Study the drawing (mm; zero at the part's minimum x, y, z) and answer. A direction names the side the tool comes from. Coordinates: 2 decimals unless noted, no trailing zeros. Write each loop counter-clockwise with the first axis right and the second up, starting at its lowest first coordinate (ties: lowest second). Pieces come first, ordered by that corner, then holes. Notation, with made-up numbers: (-14, 35.25) -> (6, 35.25) arc R21 cw to (6, 66.25) -> close; hole circle Ø2 at (37, 63.5). An arc over 180 degrees is marked (long way). Answer in a Markdown table with one row per item. Add a question column.
Item 1: Section B-B on z = 127 is taken. Write down the section's boundary in (x, y).
Item 2: Straight lines are drawn through the part: line 1 (Z direction, x = 6.5, y = 74); line 2 (Y direction, x = 48.5, z = 130). For each, find the intervals that lie inside material, in ascending order. Write a range as from..to.
Item 3: Section A-A on y = 45.5 is taken. Write down the section's boundary in (x, z), then the cut area to 3 significant figures.
Item 4: Which of the six approach directions +Z, -Z, +X, -X, +Y, -Y give full straight-line access (tool end or side, diameter ignored) to the marked faces 1, 2 and 3?
Item 5: Given pin 1 Ø6 at (y, z) = (39.5, 76) entering from -X; pin 2 Ø8 at (x, z) = (52, 139) entering from +Y, each flat-ended and moving along its own axis, determine where each tip first touches the part or whether it passes through.
Item 6: Section D-D on y = 57.5 is taken. Write down the section's boundary in (x, z), then the cut area to 3 significant figures.
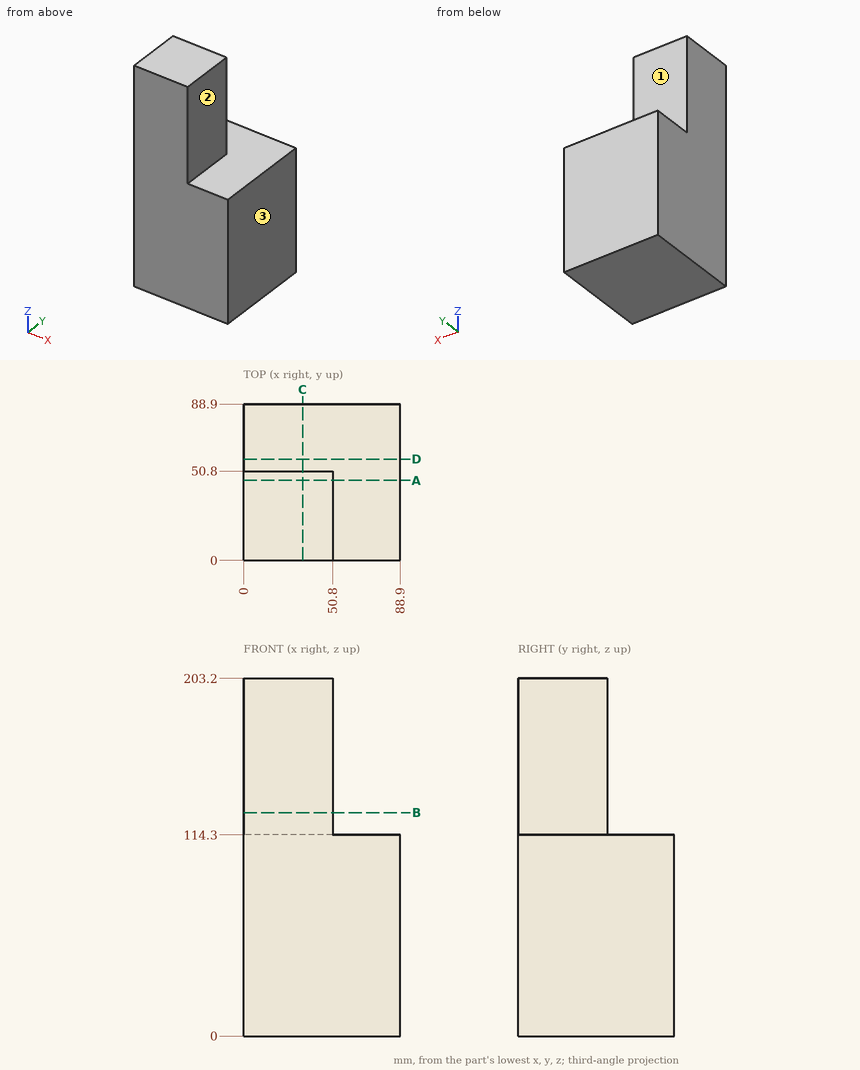
Results below:
| question | item | result |
|---|---|---|
| 1 | outline | (0, 0) -> (50.8, 0) -> (50.8, 50.8) -> (0, 50.8) -> close |
| 2 | line 1 | z = 0..114.3 |
| 2 | line 2 | y = 0..50.8 |
| 3 | outline | (0, 0) -> (88.9, 0) -> (88.9, 114.3) -> (50.8, 114.3) -> (50.8, 203.2) -> (0, 203.2) -> close |
| 3 | area | 14,700 mm2 |
| 4 | face 1 | +Z, +X, -X, +Y |
| 4 | face 2 | +Z, +X, +Y, -Y |
| 4 | face 3 | +Z, -Z, +X, +Y, -Y |
| 5 | pin 1 | stops at x = 0 |
| 5 | pin 2 | stops at y = 50.8 |
| 6 | outline | (0, 0) -> (88.9, 0) -> (88.9, 114.3) -> (0, 114.3) -> close |
| 6 | area | 10,200 mm2 |
